Part model, mm, in its own coordinate system. Face numbers are marked on the shaded views. A direction names the side the tool comes from. Round coordinates to 2 decimals unless told otherwise and drop trailing zeros. Loops run counter-clockwise (first coordinate to the right, second up) from the corner with the lowest first, then second, coordinate; pieces in that order, holes last. Notation, with made-up numbers: M 38.5,-13 L 90.5,-13 A12 cw 90.5,-3 Z; hole C 4,1 d11. An arc over 180 degrees is marked long. Write each question's results on one line, items separated by ' | '.
from build123d import *

# Parameters (mm, degrees)
F1_DEPTH = 5
F2_DEPTH = 7


with BuildPart() as f1:
    # F0 (on Front) → F1 (new body)
    with BuildSketch(Plane.XZ):
        with BuildLine():
            ThreePointArc((1, 0), (5, 4), (9, 0))
            Line((9, 0), (10, 0))
            ThreePointArc((10, 0), (5, 5), (0, 0))
            Line((0, 0), (1, 0))
        make_face()
        with BuildLine():
            Line((10, 0), (9, 0))
            ThreePointArc((9, 0), (5, -4), (1, 0))
            Line((1, 0), (0, 0))
            ThreePointArc((0, 0), (5, -5), (10, 0))
        make_face()
        with BuildLine():
            Line((10, -100), (10, 0))
            ThreePointArc((10, 0), (5, -5), (0, 0))
            Line((0, 0), (0, -100))
            ThreePointArc((0, -100), (5, -95), (10, -100))
        make_face()
        with BuildLine():
            ThreePointArc((0, -100), (5, -105), (10, -100))
            Line((10, -100), (9, -100))
            ThreePointArc((9, -100), (5, -104), (1, -100))
            Line((1, -100), (0, -100))
        make_face()
        with BuildLine():
            Line((9, -100), (10, -100))
            ThreePointArc((10, -100), (5, -95), (0, -100))
            Line((0, -100), (1, -100))
            ThreePointArc((1, -100), (5, -96), (9, -100))
        make_face()
        with BuildLine():
            ThreePointArc((1, -100), (5, -104), (9, -100))
            Line((9, -100), (1, -100))
        make_face()
        with BuildLine():
            Line((1, -100), (9, -100))
            ThreePointArc((9, -100), (5, -96), (1, -100))
        make_face()
    extrude(amount=F1_DEPTH)

    # F0 (on Front) → F2 (join)
    with BuildSketch(Plane.XZ):
        with BuildLine():
            ThreePointArc((1, -100), (5, -104), (9, -100))
            Line((9, -100), (1, -100))
        make_face()
        with BuildLine():
            Line((1, -100), (9, -100))
            ThreePointArc((9, -100), (5, -96), (1, -100))
        make_face()
    extrude(amount=-F2_DEPTH)


solid = f1.part
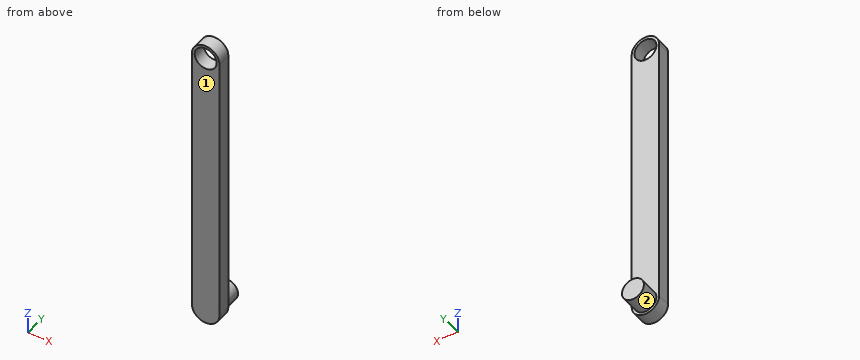
Item 1: Drop flat-ended pins along their axis: P1, Ø3, axis at x = 8.5, z = -17, coming from the +Y side; P2, Ø1.5, axis at x = 3, y = 5, coming from the -Z side; P3, Ø4, axis at x = 1.5, y = 4.5, coming from the -Z side. Give the stop position or say it passes through.
Filled sheet:
P1: y = 0 | P2: z = -103.8 | P3: z = -103.71
Item 2: Which spindle directions (+Z, -Z, +X, -X, +Y, -Y) get a long thin tool onto all of the face, cutting with end or side? Do the marked faces 1 and 2. Say none if no direction does.
Filled sheet:
face 1: +Z, -Z, +X, -X, -Y | face 2: +Y
Item 3: Band-saw the part on B-B on y = -1.25. Give the cut face in (x, z), and give its area (3 significant figures).
Filled sheet:
outline: M 0,-100 A5 ccw 10,-100 L 10,0 A5 ccw 0,0 Z; hole C 5,0 d8 | area: 1,030 mm^2
Item 4: Band-saw the part on D-D on z = -41.5. Give the cut face in (x, y).
Filled sheet:
outline: M 0,-5 L 10,-5 L 10,0 L 0,0 Z
Item 5: Band-saw the part on C-C on z = -3. Give the cut face in (x, y), and give its area (3 significant figures).
Filled sheet:
outline: M 0,-5 L 2.35,-5 L 2.35,0 L 0,0 Z; M 7.65,-5 L 10,-5 L 10,0 L 7.65,0 Z | area: 23.5 mm^2
Item 6: Wall check: L1, parallel to Z at x = 5, y = -3.75; L2, parallel to Y at x = 2.25, z = -47; L3, parallel to Z at x = 8, y = -1. Give the ranges that are in metal, low to high.
Filled sheet:
L1: -105 to -4, 4 to 5 | L2: -5 to 0 | L3: -104 to -2.65, 2.65 to 4
Item 7: Band-saw the part on A-A on x = 5. Give the cut face in (y, z), and give its area (3 significant figures).
Filled sheet:
outline: M -5,-105 L 0,-105 L 0,-104 L 7,-104 L 7,-96 L 0,-96 L 0,-4 L -5,-4 Z; M -5,4 L 0,4 L 0,5 L -5,5 Z | area: 566 mm^2
